Read the model definition and answer for the solid it produces. Units are mm, in the model's axes. Coordinates: 2 decimals unless noted, no trailing zeros. Order: outer loops, then holes, each group sorted by start corner. A loop starts at its lowest first (then second) coordinate and runs counter-clockwise, first axis right, second up. Notation, with made-up numbers: M 51,24 L 75,24 A22 cw 75,62 Z; hole C 28.5,38 d9. An arc over 180 degrees is marked long. Write each question's results on one line, items separated by ' | '.
Autodesk Inventor part; units mm, degrees
ref_plane "YZ Plane" through (0, 0, 0) normal (1, 0, 0) x (0, 1, 0)
ref_plane "XZ Plane" through (0, 0, 0) normal (0, 1, 0) x (-1, 0, 0)
ref_plane "XY Plane" through (0, 0, 0) normal (0, 0, 1) x (1, 0, 0)
sketch "Sketch1" plane through (0, 0, 0) normal (0, 1, 0) x (-1, 0, 0)
  line L0 (0, 0) -> (19.05, 0)
  line L1 (19.05, 0) -> (19.05, -152.4)
  line L2 (19.05, -152.4) -> (0, -152.4)
  line L3 (0, -152.4) -> (0, 0)
  dimension "d0" = 152.4
  dimension "d1" = 19.05
extrude "Extrusion1" add sketch "Sketch1" along normal blind 12.7
sketch "Sketch2" plane through (0, 12.7, 0) normal (0, 1, 0) x (1, 0, 0)
  line L0 (-19.05, 0) -> (0, 0)
  line L1 (-19.05, 152.4) -> (-19.05, 0)
  line L2 (0, 0) -> (-19.05, 152.4)
  line L3 (0, 0) -> (0, 152.4)
  line L4 (-19.05, 0) -> (0, 152.4)
  line L5 (-9.525, 76.2) -> (-9.525, 0)
  line L6 (-9.525, 76.2) -> (-9.525, 152.4)
  line L7 (0, 152.4) -> (-19.05, 152.4)
  circle A0 centre (-9.525, 31.8589) radius 1.7859
  circle A1 centre (-9.525, 121.157) radius 1.7859
  dimension "d4" = 3.5719
  dimension "d5" = 3.5719
extrude "Extrusion2" cut sketch "Sketch2" against normal blind 34.925 contours A0 L5 | L5 A0 | A1 L6 | L6 A1
fillet "Fillet1" radius 3.175 8 edges at (0, 6.35, 0) (-19.05, 6.35, 0) (-9.525, 0, 0) (0, 0, -76.2) (0, 6.35, -152.4) (-9.525, 0, -152.4) (-19.05, 6.35, -152.4) (-19.05, 0, -76.2)
(1) Given pin 1 (2 mm diameter, centred on x = -2, z = -50, fed in from -Y), flat-ended and moving along its own axis, determine where the tip first touches the part or whether it passes through.
Conclusion:
pin 1: y = 0
(2) The part is cut by section C-C, the plane x = -1.25. Write down the section's boundary in (y, z) (3 decimals), then the cut area to 3 significant figures.
Conclusion:
outline: M 0.65,-149.225 A2.525 ccw 3.175,-151.75 L 12.7,-151.75 L 12.7,-0.65 L 3.175,-0.65 A2.525 ccw 0.65,-3.175 Z | area: 1,820 mm²
(3) The mould has two halves that part along X. Classify faces 1 (the cylindrical face through (-0.91, 8, -151.45)), 2 (the cylindrical face through (-9.757, 6.439, -122.928)), 3 (the cylindrical face through (-18.14, 8, -0.95)): pulls with the +X half, pulls with the -X half, needs draft (parallel to the pull), parting line crosses it, or undercut.
Conclusion:
face 1: pulls with the +X half | face 2: undercut | face 3: pulls with the -X half
(4) The part is cut by section B-B, the plane y = 1.5. Write down the section's boundary in (x, z) (3 decimals).
Conclusion:
outline: M -18.572,-149.225 A2.697 ccw -15.875,-151.922 L -3.175,-151.922 A2.697 ccw -0.478,-149.225 L -0.478,-3.175 A2.697 ccw -3.175,-0.478 L -15.875,-0.478 A2.697 ccw -18.572,-3.175 Z; hole C -9.525,-121.157 d3.572; hole C -9.525,-31.859 d3.572
(5) Straight lines are drawn through the part: line 1 (Z direction, x = -15.25, y = 2.75); line 2 (Y direction, x = -16.25, z = -102); line 3 (Z direction, x = -13.5, y = 0.5). For each, find the intervals that lie inside material, in ascending order.
Conclusion:
line 1: -152.37 to -0.03 | line 2: 0.02 to 12.7 | line 3: -150.94 to -1.46
(6) The part is cut by section A-A, the plane z = -99. Write down the section's boundary in (x, y) (3 decimals).
Conclusion:
outline: M -19.05,3.175 A3.175 ccw -15.875,0 L -3.175,0 A3.175 ccw 0,3.175 L 0,12.7 L -19.05,12.7 Z
